Design review of the part built by this model. Coordinates are the model's own, in mm. A direction names the side the tool comes from. Give positions to 0.01 mm unless a question says otherwise; leave off trailing zeros. Loops run counter-clockwise (first coordinate to the right, second up) from the corner with the lowest first, then second, coordinate; pieces in that order, holes last. Notation, with made-up numbers: (23.5, 66.5) - (40.5, 66.5) arc R18 cw to (40.5, 90.5) - close; hole circle Ø5 at (-2, 44). An arc over 180 degrees is marked (long way). Write each question's results on one line, items separated by ' | '.
from build123d import *

# Parameters (mm, degrees)
F1_DEPTH = 25.4
F3_DEPTH = 25.4


with BuildPart() as f1:
    # F0 (on Right) → F1 (new body)
    with BuildSketch(Plane.YZ):
        with BuildLine():
            ThreePointArc((12.43875, -2.562713), (12.634519, -1.287998), (12.7, 0))
            ThreePointArc((12.7, 0), (12.634519, 1.287998), (12.43875, 2.562713))
            ThreePointArc((12.43875, 2.562713), (10.998523, 6.35), (8.43875, 9.490917))
            ThreePointArc((8.43875, 9.490917), (6.35, 10.998523), (4, 12.05363))
            ThreePointArc((4, 12.05363), (0, 12.7), (-4, 12.05363))
            ThreePointArc((-4, 12.05363), (-6.35, 10.998523), (-8.43875, 9.490917))
            ThreePointArc((-8.43875, 9.490917), (-10.998523, 6.35), (-12.43875, 2.562713))
            ThreePointArc((-12.43875, 2.562713), (-12.7, 0), (-12.43875, -2.562713))
            ThreePointArc((-12.43875, -2.562713), (-10.998523, -6.35), (-8.43875, -9.490917))
            ThreePointArc((-8.43875, -9.490917), (-6.35, -10.998523), (-4, -12.05363))
            ThreePointArc((-4, -12.05363), (0, -12.7), (4, -12.05363))
            ThreePointArc((4, -12.05363), (6.35, -10.998523), (8.43875, -9.490917))
            ThreePointArc((8.43875, -9.490917), (10.998523, -6.35), (12.43875, -2.562713))
        make_face()
        with BuildLine():
            ThreePointArc((8.43875, 9.490917), (10.998523, 6.35), (12.43875, 2.562713))
            Line((12.43875, 2.562713), (15.462624, 6.617949))
            Line((15.462624, 6.617949), (14.462624, 8.35))
            Line((14.462624, 8.35), (13.462624, 10.082051))
            Line((13.462624, 10.082051), (8.43875, 9.490917))
        make_face()
        with BuildLine():
            Line((15.462624, -6.617949), (12.43875, -2.562713))
            ThreePointArc((12.43875, -2.562713), (10.998523, -6.35), (8.43875, -9.490917))
            Line((8.43875, -9.490917), (13.462624, -10.082051))
            Line((13.462624, -10.082051), (14.462624, -8.35))
            Line((14.462624, -8.35), (15.462624, -6.617949))
        make_face()
        with BuildLine():
            ThreePointArc((-4, 12.05363), (0, 12.7), (4, 12.05363))
            Line((4, 12.05363), (2, 16.7))
            Line((2, 16.7), (0, 16.7))
            Line((0, 16.7), (-2, 16.7))
            Line((-2, 16.7), (-4, 12.05363))
        make_face()
        with BuildLine():
            Line((2, -16.7), (4, -12.05363))
            ThreePointArc((4, -12.05363), (0, -12.7), (-4, -12.05363))
            Line((-4, -12.05363), (-2, -16.7))
            Line((-2, -16.7), (0, -16.7))
            Line((0, -16.7), (2, -16.7))
        make_face()
        with BuildLine():
            ThreePointArc((-12.43875, 2.562713), (-10.998523, 6.35), (-8.43875, 9.490917))
            Line((-8.43875, 9.490917), (-13.462624, 10.082051))
            Line((-13.462624, 10.082051), (-14.462624, 8.35))
            Line((-14.462624, 8.35), (-15.462624, 6.617949))
            Line((-15.462624, 6.617949), (-12.43875, 2.562713))
        make_face()
        with BuildLine():
            Line((-13.462624, -10.082051), (-8.43875, -9.490917))
            ThreePointArc((-8.43875, -9.490917), (-10.998523, -6.35), (-12.43875, -2.562713))
            Line((-12.43875, -2.562713), (-15.462624, -6.617949))
            Line((-15.462624, -6.617949), (-14.462624, -8.35))
            Line((-14.462624, -8.35), (-13.462624, -10.082051))
        make_face()
    extrude(amount=F1_DEPTH)

    # F2 (on face) → F3 (cut)
    with BuildSketch(Plane.YZ.offset(25.4)):
        with BuildLine():
            ThreePointArc((2.077989, 2.300426), (0, 3.1), (-2.077989, 2.300426))
            ThreePointArc((-2.077989, 2.300426), (0, -3.1), (2.077989, 2.300426))
        make_face()
    extrude(amount=-F3_DEPTH, mode=Mode.SUBTRACT)


solid = f1.part
(1) Wall thickness on line 1 along Z through (x, y) = (19.5, 0); line 2 along Z through (x, y) = (12, 13.5); line 3 along Y through (x, z) = (9, -2): over which ranges is each line inside the solid? List them lowest first. Write a range as from..to.
Answers below:
line 1: -16.7..-3.1, 3.1..16.7 | line 2: -10.02..-3.99, 3.99..10.02 | line 3: -12.54..-2.37, 2.37..12.54
(2) Take a section at C-C on z = 14.5. Give the boundary of the cut face in (x, y).
Answers below:
outline: (0, -2.95) - (25.4, -2.95) - (25.4, 2.95) - (0, 2.95) - close
(3) Draft analysis for pull direction Y (two halves, no side actions). For faces 1 (the flat face through (12.52, 10.99, 9.79)), 2 (the flat face through (12.522, -13.972, 4.619)), 3 (the flat face through (13, 0, -16.7)), state which applies: pulls with the +Y half, pulls with the -Y half, needs draft (parallel to the pull), parting line crosses it, or undercut.
Answers below:
face 1: undercut | face 2: pulls with the -Y half | face 3: needs draft
(4) Take a section at D-D on y = 8. Give the boundary of the cut face in (x, z).
Answers below:
outline: (0, -9.86) - (25.4, -9.86) - (25.4, 9.86) - (0, 9.86) - close
(5) Insertion check: P1, Ø1.5, axis at x = 19.5, z = -8.5, coming from the -Y side; P2, Ø1.5, axis at x = 6, z = -3, coming from the -Y side; P3, Ø1.5, axis at x = 10, y = -10.5, coming from the +Z side. Each pin has a flat end and moves straight along its axis. Give the tip position at first contact, or say it passes through.
Answers below:
P1: y = -14.81 | P2: y = -13.32 | P3: z = 9.82
(6) Take a section at B-B on x = 12. Give the boundary of the cut face in (y, z), plus the area to 3 significant figures.
Answers below:
outline: (-15.46, -6.62) - (-13.46, -10.08) - (-8.44, -9.49) arc R12.7 ccw to (-4, -12.05) - (-2, -16.7) - (2, -16.7) - (4, -12.05) arc R12.7 ccw to (8.44, -9.49) - (13.46, -10.08) - (15.46, -6.62) - (12.44, -2.56) arc R12.7 ccw to (12.7, 0) arc R12.7 ccw to (12.44, 2.56) - (15.46, 6.62) - (13.46, 10.08) - (8.44, 9.49) arc R12.7 ccw to (4, 12.05) - (2, 16.7) - (-2, 16.7) - (-4, 12.05) arc R12.7 ccw to (-8.44, 9.49) - (-13.46, 10.08) - (-15.46, 6.62) - (-12.44, 2.56) arc R12.7 ccw to (-12.44, -2.56) - close; hole (-2.08, 2.3) arc R3.1 ccw (long way) to (2.08, 2.3) arc R3.1 ccw to start | area: 623 mm2
(7) Take a section at A-A on y = 0. Give the boundary of the cut face in (x, z), plus the area to 3 significant figures.
Answers below:
outline: (0, -16.7) - (25.4, -16.7) - (25.4, -3.1) - (0, -3.1) - close; (0, 3.1) - (25.4, 3.1) - (25.4, 16.7) - (0, 16.7) - close | area: 691 mm2
(8) Tool access review of faces 4 (the cylindrical face through (12.522, 6.319, -11.017)), 5 (the flat face through (12.522, 13.972, -4.619)), 6 (the flat face through (12.52, -13.93, -4.56)), 7 (the flat face through (12.522, -10.916, 9.782)): name each direction out of +Z, -Z, +X, -X, +Y, -Y from which nothing blocks a thin tool from reaching the whole face with its end or side.
Answers below:
face 4: -Z, +X, -X | face 5: +X, -X, +Y | face 6: +X, -X, -Y | face 7: +Z, +X, -X
